```python
from build123d import *

# Parameters (mm, degrees)
MODEL_4_R           = 1.725
MODEL_4_W           = 14.999999996
MODEL_4_H           = 19.999999994
BOSS_EXTRUDE3_DEPTH = 5


with BuildPart() as part:
    # Model_4 → Boss-Extrude3 (new body)
    with BuildSketch(Plane.XY):
        with BuildLine():
            Line((159.088901233, 54.770886004), (159.088901233, 42.770886007))
            Line((159.088901233, 42.770886007), (148.833688241, 42.770886007))
            add(Edge.make_bspline(
                [(148.833688241, 42.770886007), (147.703902982, 42.770886039), (146.607419644, 42.388260099), (145.722916781, 41.685359384)],
                knots=[2, 2, 2, 2, 3, 3, 3, 3], degree=3))
            Line((145.722916781, 41.685359384), (142.978129629, 39.504119451))
            add(Edge.make_bspline(
                [(142.978129629, 39.504119451), (141.78451535, 38.555572629), (141.088901059, 37.114262879), (141.088901059, 35.589646165)],
                knots=[4, 4, 4, 4, 5, 5, 5, 5], degree=3))
            Line((141.088901059, 35.589646165), (141.088901059, 21.521355488))
            Line((141.088901059, 21.521355488), (145.783498532, 26.215953035))
            Line((145.783498532, 26.215953035), (150.088901196, 21.91055044))
            Line((150.088901196, 21.91055044), (150.088901196, 7.770885671))
            Line((150.088901196, 7.770885671), (130.355887494, 7.770885671))
            add(Edge.make_bspline(
                [(130.355887494, 7.770885671), (130.178023326, 7.770885671), (130.000285852, 7.780376365), (129.823433077, 7.799317277)],
                knots=[10, 10, 10, 10, 11, 11, 11, 11], degree=3))
            Line((129.823433077, 7.799317277), (111.354083681, 9.777355295))
            add(Edge.make_bspline(
                [(111.354083681, 9.777355295), (111.177236079, 9.796295653), (111.002244565, 9.80578636), (110.8243856, 9.805786903)],
                knots=[12, 12, 12, 12, 13, 13, 13, 13], degree=3))
            add(Edge.make_bspline(
                [(110.8243856, 9.805786903), (108.600397254, 9.805793694), (93.088622023, 9.805793695)],
                knots=[13, 13, 13, 14, 14, 14], degree=2))
            Line((93.088622023, 9.805793695), (93.088622023, 17.30579417))
            Line((93.088622023, 17.30579417), (98.088808744, 17.30579417))
            Line((98.088808744, 17.30579417), (98.088808744, 32.555614676))
            add(Edge.make_bspline(
                [(98.088808744, 32.555614676), (98.088808739, 32.969898599), (98.424705306, 33.30571401), (98.838989216, 33.305613899)],
                knots=[17, 17, 17, 17, 18, 18, 18, 18], degree=3))
            Line((98.838989216, 33.305613899), (102.763713878, 33.304665432))
            add(Edge.make_bspline(
                [(102.763713878, 33.304665432), (103.071437534, 33.304591066), (103.347162069, 33.116027604), (103.458534777, 32.829165314)],
                knots=[19, 19, 19, 19, 20, 20, 20, 20], degree=3))
            add(Edge.make_bspline(
                [(103.458534777, 32.829165314), (104.256761577, 30.773175353), (106.259888758, 29.305794495), (108.589100574, 29.305794495)],
                knots=[20, 20, 20, 20, 21, 21, 21, 21], degree=3))
            Line((108.589100574, 29.305794495), (111.188773507, 29.305794495))
            add(Edge.make_bspline(
                [(111.188773507, 29.305794495), (111.741058256, 29.305794495), (112.188773507, 29.753509745), (112.188773507, 30.305794494)],
                knots=[22, 22, 22, 22, 23, 23, 23, 23], degree=3))
            Line((112.188773507, 30.305794494), (112.188773507, 39.305794492))
            add(Edge.make_bspline(
                [(112.188773507, 39.305794492), (112.188773506, 39.858079241), (111.741058256, 40.305794491), (111.188773507, 40.305794491)],
                knots=[24, 24, 24, 24, 25, 25, 25, 25], degree=3))
            Line((111.188773507, 40.305794491), (108.589100574, 40.305794491))
            add(Edge.make_bspline(
                [(108.589100574, 40.305794491), (106.259590893, 40.305794491), (104.256249253, 38.838038305), (103.458228599, 36.781634874)],
                knots=[26, 26, 26, 26, 27, 27, 27, 27], degree=3))
            add(Edge.make_bspline(
                [(103.458228599, 36.781634874), (103.346863397, 36.494660115), (103.071039563, 36.306024593), (102.763213768, 36.306010412)],
                knots=[27, 27, 27, 27, 28, 28, 28, 28], degree=3))
            Line((102.763213768, 36.306010412), (98.838842522, 36.30582961))
            add(Edge.make_bspline(
                [(98.838842522, 36.30582961), (98.424615889, 36.305810532), (98.088808739, 36.64160222), (98.088808744, 37.055828853)],
                knots=[29, 29, 29, 29, 30, 30, 30, 30], degree=3))
            Line((98.088808744, 37.055828853), (98.088808744, 52.295139183))
            Line((98.088808744, 52.295139183), (93.088622023, 52.295139183))
            Line((93.088622023, 52.295139183), (93.088622023, 59.795139659))
            Line((93.088622023, 59.795139659), (116.088583489, 59.795139659))
            add(Edge.make_bspline(
                [(116.088583489, 59.795139659), (117.188583796, 59.795139659), (118.724980283, 59.158743333), (119.502797904, 58.380925601)],
                knots=[34, 34, 34, 34, 35, 35, 35, 35], degree=3))
            Line((119.502797904, 58.380925601), (121.67437012, 56.209353091))
            add(Edge.make_bspline(
                [(121.67437012, 56.209353091), (122.452187569, 55.431535532), (123.988583716, 54.795139347), (125.08858378, 54.795139347)],
                knots=[36, 36, 36, 36, 37, 37, 37, 37], degree=3))
            Line((125.08858378, 54.795139347), (159.088901233, 54.770886004))
        make_face()
        with Locations((154.813901136, 48.770885771)):
            Circle(MODEL_4_R, mode=Mode.SUBTRACT)
        with Locations((126.592244968, 32.300466217)):
            Rectangle(MODEL_4_W, MODEL_4_H, mode=Mode.SUBTRACT)
    extrude(amount=BOSS_EXTRUDE3_DEPTH)


solid = part.part
```
Read the model definition and answer for the solid it produces. Units are mm, in the model's axes. A direction names the side the tool comes from. Round coordinates to 2 decimals unless told otherwise and drop trailing zeros. Loops run counter-clockwise (first coordinate to the right, second up) from the corner with the lowest first, then second, coordinate; pieces in that order, holes last. Notation, with made-up numbers: (-40, 25) -> (-25, 25) arc R31 ccw to (-25, 61) -> close; hole circle Ø11 at (-18, -5.5). An arc over 180 degrees is marked (long way). One line per item, written item: value.
1) A cutting plane is placed at A-A (x = 154). Determine the outline of the cut face in (y, z), and give its area (3 significant figures).
Answer list:
outline: (42.77, 0) -> (47.25, 0) -> (47.25, 5) -> (42.77, 5) -> close; (50.29, 0) -> (54.77, 0) -> (54.77, 5) -> (50.29, 5) -> close
area: 44.8 mm²
2) For faces 5 (the face through (104, 59.795, 2)), 6 (the face through (148, 24, 2)), 7 (the face through (134.092, 32, 2)), 8 (the face through (96, 17.306, 2)), determine the directions among +Z, -Z, +X, -X, +Y, -Y from which every point of the face is accessible in a straight line to the end or side of a thin tool.
Answer list:
face 5: +Z, -Z, +X, -X, +Y
face 6: +Z, -Z, +X
face 7: +Z, -Z
face 8: +Z, -Z, -X
3) A cutting plane is placed at D-D (y = 57). Determine the outline of the cut face in (x, z).
Answer list:
outline: (93.09, 0) -> (120.88, 0) -> (120.88, 5) -> (93.09, 5) -> close
4) Flat-ended cylindrical pins translate along their axes: P1, Ø2, axis at x = 133.5, z = 3.5, coming from the +Y side; P2, Ø1.5, axis at x = 127, z = 3, coming from the -Y side; P3, Ø10, axis at x = 132, y = 32, coming from the +Z side; P4, Ø2.5, axis at y = 27, z = 2.5, coming from the -X side. Find the tip coordinate at first contact, or state that the pin passes through.
Answer list:
P1: stops at y = 54.79
P2: stops at y = 8.02
P3: stops at z = 5
P4: stops at x = 98.09
5) The mould has two halves that part along X. Classify faces 1 (the face through (144.37, 40.61, 2.46)), 2 (the face through (93.089, 56, 2)), 3 (the face through (119.092, 32, 2)), 4 (the face through (112.189, 35, 2)): pulls with the +X half, pulls with the -X half, needs draft (parallel to the pull), parting line crosses it, or undercut.
Answer list:
face 1: pulls with the +X half
face 2: pulls with the -X half
face 3: undercut
face 4: undercut
6) A cutting plane is placed at B-B (y = 45). Determine the outline of the cut face in (x, z).
Answer list:
outline: (98.09, 0) -> (159.09, 0) -> (159.09, 5) -> (98.09, 5) -> close
7) Consider L1, parallel to Y at x = 109, z = 0.55; L2, parallel to X at y = 39.5, z = 0.95; L3, parallel to X at y = 16.5, z = 3.45. Determine where each line is inside the solid, lowest interval first. Write a range as [from, to].
Answer list:
L1: y = [9.81, 29.31], [40.31, 59.8]
L2: x = [98.09, 105.73], [112.17, 119.09], [134.09, 142.97]
L3: x = [93.09, 150.09]
8) A cutting plane is placed at C-C (z = 1.1). Give the number of separate pieces and of enclosed holes in the cut face, and give its area (3 significant figures).
Answer list:
separate pieces: 1
enclosed holes: 2
area: 2,130 mm²
